```python
from build123d import *

# Parameters (mm, degrees)
SKETCH1_R           = 0.5
BOSS_EXTRUDE1_DEPTH = 4
CUT_EXTRUDE1_DEPTH  = 3
FILLET1_R           = 0.2


with BuildPart() as part:
    # Sketch1 → Boss-Extrude1 (new body)
    with BuildSketch(Plane(origin=(0, 0, 0), x_dir=(1, 0, 0), z_dir=(0, 1, 0))):
        Polygon((2.320929304, 2.619787619), (3.990706765, 2.754585991), (3.272556849, 1.241117105), (4.813715291, 0.584490857), (3.474481059, -0.421878381), (4.533959656, -1.719504088), (2.880443531, -1.988226614), (3.215528503, -3.629581369), (1.626531102, -3.09909609), (1.160458522, -4.708165299), (0, -3.5), (-1.160458522, -4.708165299), (-1.626531102, -3.09909609), (-3.215528503, -3.629581369), (-2.880443531, -1.988226614), (-4.533959656, -1.719504088), (-3.474481059, -0.421878381), (-4.813715291, 0.584490857), (-3.272556849, 1.241117105), (-3.990706765, 2.754585991), (-2.320929304, 2.619787619), (-2.253475412, 4.293638671), (-0.837604825, 3.398296361), (0, 4.849070475), (0.837604825, 3.398296361), (2.253475412, 4.293638671), align=None)
        with Locations(Location((0, 0, 0), (0, 0, 270))):
            Circle(SKETCH1_R, mode=Mode.SUBTRACT)
    extrude(amount=BOSS_EXTRUDE1_DEPTH)

    # Sketch2 → Cut-Extrude1 (cut)
    with BuildSketch(Plane.XZ):
        Polygon((-2.356515562, -0.355187571), (-2.394012407, -0.73845503), (-2.147128813, -1.03400274), (-2.069989712, -1.411295089), (-1.746960246, -1.620942227), (-1.562039347, -1.958735387), (-1.191566595, -2.063853884), (-0.915294931, -2.332133449), (-0.530297023, -2.323383066), (-0.187222544, -2.49831122), (0.178091766, -2.376469467), (0.557485388, -2.442503076), (0.870656321, -2.218396127), (1.252658297, -2.169667815), (1.485859241, -1.863208555), (1.836527019, -1.704048047), (1.969037046, -1.342466727), (2.257212255, -1.087016131), (2.27725727, -0.702440839), (2.477334277, -0.373398063), (2.383133191, 0), (2.477334277, 0.373398063), (2.27725727, 0.702440839), (2.257212255, 1.087016131), (1.969037046, 1.342466727), (1.836527019, 1.704048047), (1.485859241, 1.863208555), (1.252658297, 2.169667815), (0.870656321, 2.218396127), (0.557485388, 2.442503076), (0.178091766, 2.376469467), (-0.187222544, 2.49831122), (-0.530297023, 2.323383066), (-0.915294931, 2.332133449), (-1.191566595, 2.063853884), (-1.562039347, 1.958735387), (-1.746960246, 1.620942227), (-2.069989712, 1.411295089), (-2.147128813, 1.03400274), (-2.394012407, 0.73845503), (-2.356515562, 0.355187571), (-2.505316594, 0), align=None)
    extrude(amount=-CUT_EXTRUDE1_DEPTH, mode=Mode.SUBTRACT)

    # Fillet1
    fillet1_edges = [part.edges().sort_by_distance(p)[0] for p in [
        (4.813715291, 2, -0.584490857),
        (4.533959656, 2, 1.719504088),
        (3.215528503, 2, 3.629581369),
        (1.160458522, 2, 4.708165299),
        (-1.160458522, 2, 4.708165299),
        (-3.215528503, 2, 3.629581369),
        (-4.533959656, 2, 1.719504088),
        (-4.813715291, 2, -0.584490857),
        (-3.990706765, 2, -2.754585991),
        (-2.253475412, 2, -4.293638671),
        (0, 2, -4.849070475),
        (2.253475412, 2, -4.293638671),
        (3.990706765, 2, -2.754585991),
    ]]
    fillet(fillet1_edges, radius=FILLET1_R)


solid = part.part
```
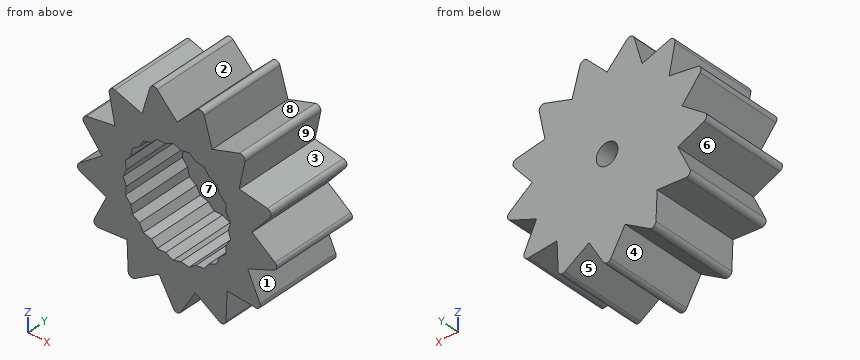
The listing builds one solid part. Answer for the finished solid, in the listing's coordinates (mm). Face numbers are marked on the shaded views. A direction names the side the tool comes from. Give positions to 0.01 mm unless a question says otherwise; leave off trailing zeros. Order: outer loops, then holes, each group sorted by start corner. A loop starts at its lowest first (then second) coordinate and runs counter-clockwise, first axis right, second up.
Item 1: Which of the six approach directions +Z, -Z, +X, -X, +Y, -Y give full straight-line access (tool end or side, diameter ignored) to the marked faces 5, 6, 7, 8 and 9?
From the geometry:
face 5: -Z, +Y, -Y
face 6: -X, +Y, -Y
face 7: -Y
face 8: +Z, +Y, -Y
face 9: +X, +Y, -Y
Item 2: For a pull along Z with two mould halves and no side action, classify the marked faces 1, 2, 3 and 4 as pulls with the +Z half, pulls with the -Z half, needs draft (parallel to the pull), parting line crosses it, or undercut.
From the geometry:
face 1: undercut
face 2: pulls with the +Z half
face 3: undercut
face 4: pulls with the -Z half
Item 3: Given pin 1 Ø1.5 at (x, z) = (-0.5, -1) entering from -Y; pin 2 Ø2 at (x, y) = (0, 0.5) entering from +Z; pin 3 Ø1 at (x, y) = (-2, 2.5) entering from -Z, each flat-ended and moving along its own axis, determine where each tip first touches the part or whether it passes through.
From the geometry:
pin 1: stops at y = 3
pin 2: stops at z = 4.51
pin 3: stops at z = -4.14
Item 4: Find the intervals of material crossed by probe 1 along Y at (x, z) = (1, -0.25); probe 2 along X at (y, z) = (3.3, 0); probe 3 along Z at (x, y) = (3.75, 2.75), in increasing order.
From the geometry:
probe 1: y = 3 to 4
probe 2: x = -4.04 to -0.5, 0.5 to 4.04
probe 3: z = -2.71 to -2.25, -1.04 to 0.21, 0.76 to 1.85
Item 5: The part is cut by section A-A, the plane z = -3.75. Give the vertices of the cut face in (x, y), and give its area (3 significant figures).
From the geometry:
outline: (-2.28, 0) - (-1.39, 0) - (-1.39, 4) - (-2.28, 4) - close; (-0.63, 0) - (0.63, 0) - (0.63, 4) - (-0.63, 4) - close; (1.39, 0) - (2.28, 0) - (2.28, 4) - (1.39, 4) - close
area: 12.1 mm2
